Verification items for the finished model (mm, model axes). A direction names the side the tool comes from. Give positions to 0.01 mm unless a question says otherwise; leave off trailing zeros. Order: outer loops, then holes, each group sorted by start corner. A loop starts at its lowest first (then second) coordinate and runs counter-clockwise, first axis right, second up. Notation, with made-up numbers: (18, 46) -> (57, 46) arc R19 ccw to (57, 51) -> close; hole circle Ø11 at (78.25, 83.25). An arc over 180 degrees is marked (long way). Return JSON: item names as keys, results as strings. Group by question number.
(1) Thickness scan on line 1 along X through (y, z) = (24, 10.25); line 2 along Z through (x, y) = (-27.1, 35); line 3 along X through (y, z) = (-1.05, 15). Record the ranges inside material, lowest first.
(2) Tool access check on faces 1 (the face through (-27.5, 37.4, 13.2)), 2 (the face through (0, 0, 11)). Record the directions out of +Z, -Z, +X, -X, +Y, -Y that give a thin tool (end or side, any length) a straight path to the whole face; none if there is none.
(3) Cross-section at B-B on z = 15. Enter the section's corners in (x, y).
(4) Cross-section at C-C on y = 35. Enter the section's corners in (x, z), then the cut area to 3 significant figures.
(5) Cross-section at A-A on x = 0. Enter the section's corners in (y, z), then the cut area to 3 significant figures.
(6) Release check for a two-part mould opening along X. For faces 3 (the face through (-0.1, -0.4, 30)), 4 (the face through (26.75, 25, 15)), 5 (the face through (28.25, 24, 15)) record: pulls with the +X half, pulls with the -X half, needs draft (parallel to the pull), parting line crosses it, or undercut.
(7) Cross-section at D-D on y = 17.5. Enter the section's corners in (x, z).
(8) Depth check by flat-ended pin: pin 1 Ø4 at (x, z) = (-19, 21.5) entering from +Y; pin 2 Ø9.5 at (y, z) = (35, 15) entering from -X. Enter the tip coordinate at first touch or a pass-through.
from build123d import *

# Parameters (mm, degrees)
BOSS_EXTRUDE1_DEPTH = 30
SKETCH3_R           = 3
CUT_EXTRUDE1_DEPTH  = 60
CUT_EXTRUDE2_REACH  = 66.792
SKETCH4_R           = 3


with BuildPart() as part:
    # Sketch2 → Boss-Extrude1 (new body)
    with BuildSketch(Plane.XY):
        Polygon((26.75, 0), (-26.75, 0), (-26.75, 50), (-28.25, 50), (-28.25, -1.5), (28.25, -1.5), (28.25, 50), (26.75, 50), align=None)
    extrude(amount=BOSS_EXTRUDE1_DEPTH)

    # Sketch3 → Cut-Extrude1 (cut)
    with BuildSketch(Plane.ZY.offset(28.25)):
        with Locations(Location((15, 35, 0), (0, 0, 270))):
            Circle(SKETCH3_R)
    extrude(amount=-CUT_EXTRUDE1_DEPTH, mode=Mode.SUBTRACT)

    # Sketch4 → Cut-Extrude2 (cut, up to next)
    with BuildSketch(Plane(origin=(0, 0, 0), x_dir=(1, 0, 0), z_dir=(0, 1, 0)), mode=Mode.PRIVATE) as cut_extrude2_sk1:
        with Locations(Location((0, -15, 0), (0, 0, 270))):
            Circle(SKETCH4_R)
    cut_extrude2_tool1 = extrude(cut_extrude2_sk1.sketch, amount=-CUT_EXTRUDE2_REACH, mode=Mode.PRIVATE) & part.part
    add(cut_extrude2_tool1.solids().sort_by_distance((0, 0, 15))[0], mode=Mode.SUBTRACT)


solid = part.part
Verdict:
{
 "1": {"line 1": "-28.25 to -26.75, 26.75 to 28.25", "line 2": "0 to 12, 18 to 30", "line 3": "-28.25 to -3, 3 to 28.25"},
 "2": {"face 1": "+X, -X", "face 2": "+Z, -Z, +Y"},
 "3": {"outline": "(-28.25, -1.5) -> (-3, -1.5) -> (-3, 0) -> (-26.75, 0) -> (-26.75, 32) -> (-28.25, 32) -> close; (-28.25, 38) -> (-26.75, 38) -> (-26.75, 50) -> (-28.25, 50) -> close; (3, -1.5) -> (28.25, -1.5) -> (28.25, 32) -> (26.75, 32) -> (26.75, 0) -> (3, 0) -> close; (26.75, 38) -> (28.25, 38) -> (28.25, 50) -> (26.75, 50) -> close"},
 "4": {"outline": "(-28.25, 0) -> (-26.75, 0) -> (-26.75, 12) -> (-28.25, 12) -> close; (-28.25, 18) -> (-26.75, 18) -> (-26.75, 30) -> (-28.25, 30) -> close; (26.75, 0) -> (28.25, 0) -> (28.25, 12) -> (26.75, 12) -> close; (26.75, 18) -> (28.25, 18) -> (28.25, 30) -> (26.75, 30) -> close", "area": "72.0 mm²"},
 "5": {"outline": "(-1.5, 0) -> (0, 0) -> (0, 12) -> (-1.5, 12) -> close; (-1.5, 18) -> (0, 18) -> (0, 30) -> (-1.5, 30) -> close", "area": "36.0 mm²"},
 "6": {"face 3": "needs draft", "face 4": "undercut", "face 5": "pulls with the +X half"},
 "7": {"outline": "(-28.25, 0) -> (-26.75, 0) -> (-26.75, 30) -> (-28.25, 30) -> close; (26.75, 0) -> (28.25, 0) -> (28.25, 30) -> (26.75, 30) -> close"},
 "8": {"pin 1": "y = 0", "pin 2": "x = -28.25"}
}
